Here's how the part is built. I have some questions about the finished solid (model axes, mm). Face numbers are marked on the shaded views. A direction names the side the tool comes from. Round coordinates to 2 decimals unless told otherwise and drop trailing zeros. Loops run counter-clockwise (first coordinate to the right, second up) from the corner with the lowest first, then second, coordinate; pieces in that order, holes last. Notation, with made-up numbers: (50, 83.25) -> (61, 83.25) arc R28 ccw to (61, 115.25) -> close; hole circle Ø6 at (-21.5, -8.75). An arc over 180 degrees is marked (long way). Use CSV: the item, a comma, the result in double quotes. Start each with the question number.
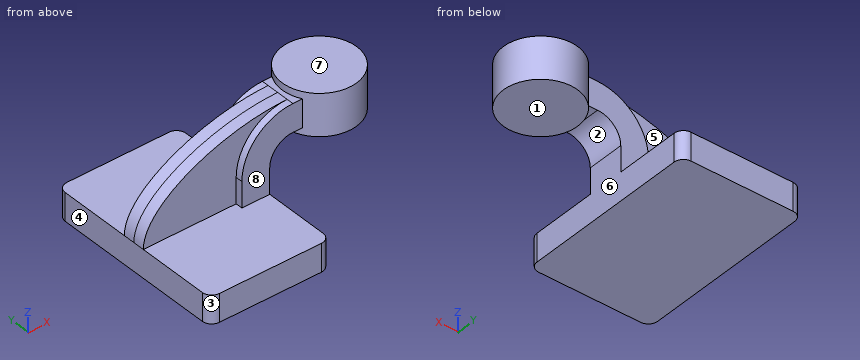
from build123d import *

# Parameters (mm, degrees)
F1_DEPTH = 63.5
F0_W     = 25.4
F0_H     = 19.05
F2_DEPTH = 12.7
F3_DEPTH = 7.9375
F5_R     = 6.35


with BuildPart() as f1:
    # F0 (on Front) → F1 (new body, symmetric)
    with BuildSketch(Plane.XZ):
        Polygon((41.275, -9.525), (41.275, 9.525), (22.225, 9.525), (-41.275, 9.525), (-41.275, -9.525), align=None)
    extrude(amount=F1_DEPTH, both=True)



with BuildPart() as f2:
    # F0 (on Front) → F2 (new body, symmetric)
    with BuildSketch(Plane.XZ):
        with Locations((73.025, 52.4002)):
            Rectangle(F0_W, F0_H)
        with BuildLine():
            Line((22.225, 9.525), (41.275, 9.525))
            Line((41.275, 9.525), (41.275, 27.0002))
            ThreePointArc((41.275, 27.0002), (45.9246798487, 38.2255201513), (57.15, 42.8752))
            Line((57.15, 42.8752), (60.325, 42.8752))
            Line((60.325, 42.8752), (60.325, 61.9252))
            Line((60.325, 61.9252), (57.15, 61.9252))
            ThreePointArc((57.15, 61.9252), (32.4542956671, 51.6959043329), (22.225, 27.0002))
            Line((22.225, 27.0002), (22.225, 9.525))
        make_face()
    extrude(amount=F2_DEPTH, both=True)


with BuildPart() as f1_1:
    add(f1.part)

    add(f2.part)  # F3 merges F2
    # F0 (on Front) → F3 (join, symmetric)
    with BuildSketch(Plane.XZ):
        with BuildLine():
            Line((-41.275, 9.525), (22.225, 9.525))
            Line((22.225, 9.525), (22.225, 27.0002))
            ThreePointArc((22.225, 27.0002), (32.4542956671, 51.6959043329), (57.15, 61.9252))
            add(Edge.make_bspline(
                [(-41.275, 9.525), (-41.1560833454, 37.1647924185), (10.9962709248, 61.9252), (57.15, 61.9252)],
                knots=[0, 0, 0, 0, 111.5045361635, 111.5045361635, 111.5045361635, 111.5045361635], degree=3))
        make_face()
    extrude(amount=F3_DEPTH, both=True)

    # F0 (on Front) → F4 (revolve)
    with BuildSketch(Plane.XZ):
        Polygon((85.725, 61.9252), (85.725, 42.8752), (85.725, 38.1), (111.125, 38.1), (111.125, 66.675), (85.725, 66.675), align=None)
    revolve(axis=Axis((85.725, 0, 52.3875), (0, 0, 1)))

    # F5
    f5_edges = [f1_1.edges().sort_by_distance(p)[0] for p in [
        (-41.275, -63.5, 0),
        (41.275, -63.5, 0),
        (41.275, 63.5, 0),
        (-41.275, 63.5, 0),
    ]]
    fillet(f5_edges, radius=F5_R)


solid = f1_1.part
Q1. For the marked faces 4, 5, 6, 7 and 8, which set-ups out of +Z, -Z, +X, -X, +Y, -Y let a thin tool reach every point of the face, with its end or its side?
Q2. I want a section at C-C, the plane y = 39.5. List the corners of the cut face in (x, z) for me (3 decimals).
Q3. Will these pins go through, and if not, where does the flat tip stop? pin 1 Ø18.5 at (y, z) = (19.5, 7) entering from +X (3 decimals); pin 2 Ø4 at (x, y) = (83, -10) entering from -Z; pin 3 Ø6 at (x, z) = (-14.5, 45.5) entering from -Y; pin 4 Ø3.5 at (x, y) = (59.5, -4.5) entering from +Z (3 decimals).
Q4. I need wall thicknesses on line 1 along X through (y, z) = (-7, 6) (3 decimals); line 2 along Z through (x, y) = (99.5, -9) (3 decimals); line 3 along Y through (x, z) = (-24, 28.5). Which ranges of each line are inside material? Lowest first, please.
Q5. I want a section at A-A, the plane y = 23. List the corners of the cut face in (x, z) for me (3 decimals).
Q6. I want a section at D-D, the plane x = 82.5. List the corners of the cut face in (y, z) for me (3 decimals), then the cut area to 3 significant figures.
Q7. I want a section at B-B, the plane z = -0.5. List the corners of the cut face in (x, y) for me (3 decimals), then the cut area to 3 significant figures.
Q8. If we mould it in two halves opening along X, with no side actions, what happens to the marked faces 1, 2 and 3? For each: pulls with the +X half, pulls with the -X half, needs draft (parallel to the pull), parting line crosses it, or undercut.
Values found:
1,face 4,"+Z, -Z, -X, +Y, -Y"
1,face 5,"+Z, -X, +Y"
1,face 6,"-Z, +X, +Y, -Y"
1,face 7,"+Z, +X, -X, +Y, -Y"
1,face 8,"+Z, -X, -Y"
2,outline,"(-41.275, -9.525) -> (41.275, -9.525) -> (41.275, 9.525) -> (-41.275, 9.525) -> close"
3,pin 1,"x = 41.275"
3,pin 2,"z = 38.1"
3,pin 3,"y = -7.94"
3,pin 4,"z = 66.675"
4,line 1,"-41.275 to 41.275"
4,line 2,"38.1 to 66.675"
4,line 3,"-7.94 to 7.94"
5,outline,"(-41.275, -9.525) -> (41.275, -9.525) -> (41.275, 9.525) -> (-41.275, 9.525) -> close; (74.947, 38.1) -> (96.503, 38.1) -> (96.503, 66.675) -> (74.947, 66.675) -> close"
6,outline,"(-25.194, 38.1) -> (25.194, 38.1) -> (25.194, 66.675) -> (-25.194, 66.675) -> close"
6,area,"1,440 mm2"
7,outline,"(-41.275, -57.15) arc R6.35 ccw to (-34.925, -63.5) -> (34.925, -63.5) arc R6.35 ccw to (41.275, -57.15) -> (41.275, 57.15) arc R6.35 ccw to (34.925, 63.5) -> (-34.925, 63.5) arc R6.35 ccw to (-41.275, 57.15) -> close"
7,area,"10,400 mm2"
8,face 1,"needs draft"
8,face 2,"undercut"
8,face 3,"pulls with the -X half"
